Autodesk Inventor part; units mm, degrees
ref_plane "Work Plane1" through (0, 33, 2) normal (1, 0, 0) x (0, 0, -1)
ref_plane "YZ Plane" through (0, 0, 0) normal (1, 0, 0) x (0, 1, 0)
ref_plane "XZ Plane" through (0, 0, 0) normal (0, 1, 0) x (-1, 0, 0)
sketch "Sketch1" plane through (0, 0, 0) normal (0, 0, 1) x (1, 0, 0)
  line L0 (-31, -31) -> (31, -31)
  line L1 (31, -31) -> (31, 31)
  line L2 (31, 31) -> (-31, 31)
  line L3 (-31, 31) -> (-31, -31)
  line L4 (-31, -31) -> (31, 31) construction
  line L5 (31, -31) -> (-31, 31) construction
  line L6 (-33, 33) -> (33, 33)
  line L7 (33, 33) -> (33, -33)
  line L8 (33, -33) -> (-33, -33)
  line L9 (-33, -33) -> (-33, 33)
  point P0 (0, 0)
  dimension "d0" = 62
  dimension "d1" = 62
  dimension "d2" = 2
extrude "Extrusion1" add sketch "Sketch1" along normal blind 2 contours L3 L2 L1 L0 | L6 L7 L8 L9
extrude "Extrusion2" add sketch "Sketch1" against normal blind 12
sketch "Sketch2" plane through (-33, 33, 2) normal (0, 1, 0) x (1, 0, 0)
  line L0 (8, 3) -> (58, 3)
  line L1 (58, 3) -> (58, 0)
  line L2 (58, 0) -> (8, 0)
  line L3 (8, 0) -> (8, 3)
  line L4 (0, 14) -> (0, 0)
  line L5 (0, 14) -> (66, 14)
  point P0 (33, 2)
  dimension "d7" = 50
  dimension "d8" = 3
  dimension "d9" = 8
  dimension "d10" = 11
extrude "Extrusion3" add sketch "Sketch2" along normal blind 12
sketch "Sketch3" plane through (25, 33, -1) normal (0, 0, -1) x (-1, 0, 0)
  line L0 (50, 12) -> (0, 12)
  line L1 (50, 0) -> (50, 12)
  line L2 (0, 12) -> (50, 12)
  line L3 (50, 12) -> (50, 9)
  line L4 (50, 9) -> (0, 9)
  line L5 (0, 9) -> (0, 12)
  point P0 (25, -33)
  dimension "d13" = 3
extrude "Extrusion4" add sketch "Sketch3" along normal blind 60
sketch "Sketch8" plane through (-25, 33, -1) normal (-1, 0, 0) x (0, 0, 1)
  line L0 (0, 9) -> (-60, 9)
  line L1 (0, 9) -> (-60, 9)
  line L2 (-60, 9) -> (-60, 0)
  line L3 (-60, 0) -> (0, 0)
  line L4 (0, 0) -> (0, 9)
  line L5 (-60, 9) -> (-10.9892, 0)
  point P0 (1, -33)
  dimension "d43" = 9
extrude "Extrusion9" add sketch "Sketch8" against normal blind 2 contours L4 L3 L5 L0
ref_plane "Work Plane1" through (0, 33, 2) normal (1, 0, 0) x (0, 0, -1)
mirror "Mirror1" about plane through (0, 33, 2) normal (1, 0, 0) of "Extrusion9"
sketch "Sketch9" plane through (-33, 45, 2) normal (0, 1, 0) x (1, 0, 0)
  circle A0 centre (33, 45) radius 5.5
  circle A1 centre (33, 45) radius 6.45
  circle A2 centre (14.625, 45) radius 2.125
  circle A3 centre (51.375, 45) radius 2.125
  line L0 (14.279, 47.0966) -> (28.2925, 49.4093)
  line L1 (14.2406, 42.9101) -> (28.6201, 40.2652)
  line L2 (51.7217, 47.0965) -> (37.702, 49.4152)
  line L3 (51.7594, 42.9101) -> (37.3799, 40.2652)
  line L4 (33, 45) -> (51.375, 45)
  line L5 (33, 45) -> (14.625, 45)
  circle A4 centre (18.825, 40.6) radius 1.15
  circle A5 centre (47.175, 49.4) radius 1.15
  circle A6 centre (47.175, 45.2183) radius 1.15
  circle A7 centre (18.825, 49.4) radius 1.15
  circle A8 centre (28.6, 30.825) radius 1.15
  circle A9 centre (37.4, 30.825) radius 1.15
  circle A10 centre (32.7817, 59.175) radius 1.15
  circle A11 centre (28.6, 59.175) radius 1.15
  circle A12 centre (47.175, 40.6) radius 1.15
  circle A13 centre (47.175, 49.4) radius 1.15
  circle A14 centre (18.825, 44.7817) radius 1.15
  circle A15 centre (18.825, 40.6) radius 1.15
  circle A16 centre (37.4, 59.175) radius 1.15
  circle A17 centre (28.6, 59.175) radius 1.15
  circle A18 centre (33.2183, 30.825) radius 1.15
  circle A19 centre (37.4, 30.825) radius 1.15
  line L6 (8, 0) -> (58, 0)
  line L7 (8, 0) -> (8, 63)
  point P0 (33, 2)
  point P1 (7.2363, 31.7405)
  point P2 (37.6183, 45)
  dimension "d48" = 12.9
  dimension "d49" = 4.25
  dimension "d50" = 4.25
  dimension "d51" = 9.15
  dimension "d52" = 9.15
  dimension "d53" = 41
  dimension "d54" = 18.375
  dimension "d55" = 2.3
  dimension "d56" = 4.4
  dimension "d57" = 4.2
  dimension "d58" = 2.3
  dimension "d59" = 4.4
  dimension "d60" = 4.2
  dimension "d62" = 360
  dimension "d64" = 45
  dimension "d67" = 25
extrude "Extrusion10" cut sketch "Sketch9" against normal blind 10 contours A4 | A5 | A7 | A8 | A9 | A11 | A12 | A16
extrude "Extrusion11" cut sketch "Sketch9" against normal blind 10 contours L4 L5 A0 | A0 L5 L4
properties part number "pan_base_holder_third"
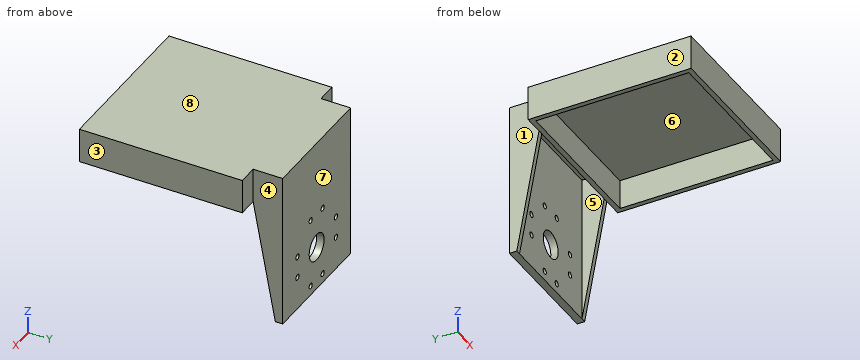
Work out the finished part from the listing and answer in its coordinate system (mm). Face numbers are marked on the shaded views. A direction names the side the tool comes from. Coordinates: 2 decimals unless noted, no trailing zeros. Write each loop counter-clockwise with the first axis right and the second up, starting at its lowest first coordinate (ties: lowest second). Pieces come first, ordered by that corner, then holes.
Q1. Which of the six approach directions +Z, -Z, +X, -X, +Y, -Y give full straight-line access (tool end or side, diameter ignored) to the marked faces 1, 2, 3, 4 and 5?
Q2. Each of these flat-tipped pins is pushed along its axis until it touches: pin 1 Ø2 at (x, z) = (4.4, -57.175) entering from +Y; pin 2 Ø2 at (x, y) = (24.5, 9) entering from -Z; pin 3 Ø9.5 at (y, z) = (39.5, -39) entering from +X; pin 4 Ø13 at (y, z) = (41, -27.5) entering from -X. Where does it stop, or does it pass through?
Q3. Find the intervals of material crossed by line 1 (Z direction, x = 0, y = 43); line 2 (Y direction, x = 29, z = -11); line 3 (X direction, y = 43.6, z = -47.4) (3 decimals), in increasing order.
Q4. A cutting plane is placed at A-A, the plane x = 0. Give the vertices of the cut face in (y, z), then the cut area to 3 significant figures.
Q5. A cutting plane is placed at C-C, the plane x = -19. Give the vertices of the cut face in (y, z).
Q6. Determine the mould class of the marked faces 6, 7 and 8 for opening direction Y: released by +Y, released by -Y, zero draft, split by the parting line, or undercut.
Q7. A cutting plane is placed at D-D, the plane z = -43. Give the vertices of the cut face in (x, y), then the cut area to 3 significant figures.
Q8. A cutting plane is placed at B-B, the plane y = -11. Give the vertices of the cut face in (x, z).
Findings below:
1. face 1: +Z, -Z, -X, +Y
1. face 2: +Z, -Z, -X, +Y, -Y
1. face 3: +Z, -Z, +X, +Y, -Y
1. face 4: +Z, -Z, +X, +Y
1. face 5: -Z
2. pin 1: passes through
2. pin 2: stops at z = 0
2. pin 3: stops at x = 25
2. pin 4: stops at x = -25
3. line 1: z = -61 to -48.5, -37.5 to 2
3. line 2: y = -33 to -31, 31 to 33
3. line 3: x = -25 to -15.325, -13.025 to -3.3, 3.3 to 13.025, 15.325 to 25
4. outline: (-33, -12) - (-31, -12) - (-31, 0) - (31, 0) - (31, -12) - (33, -12) - (33, -1) - (42, -1) - (42, -37.5) - (45, -37.5) - (45, 2) - (-33, 2) - close; (42, -61) - (45, -61) - (45, -48.5) - (42, -48.5) - close
4. area: 363 mm2
5. outline: (-33, -12) - (-31, -12) - (-31, 0) - (31, 0) - (31, -12) - (33, -12) - (33, -1) - (42, -1) - (42, -61) - (45, -61) - (45, 2) - (-33, 2) - close
6. face 6: undercut
6. face 7: released by +Y
6. face 8: zero draft
7. outline: (-25, 38.69) - (-23, 38.69) - (-23, 42) - (-5.5, 42) - (-5.5, 45) - (-25, 45) - close; (5.5, 42) - (23, 42) - (23, 38.69) - (25, 38.69) - (25, 45) - (5.5, 45) - close
7. area: 130 mm2
8. outline: (-33, -12) - (-31, -12) - (-31, 0) - (31, 0) - (31, -12) - (33, -12) - (33, 2) - (-33, 2) - close
